Autodesk Inventor part; units mm, degrees
ref_plane "YZ Plane" through (0, 0, 0) normal (1, 0, 0) x (0, 1, 0)
ref_plane "XZ Plane" through (0, 0, 0) normal (0, 1, 0) x (-1, 0, 0)
ref_plane "XY Plane" through (0, 0, 0) normal (0, 0, 1) x (1, 0, 0)
sketch "Sketch1" plane through (0, 0, 0) normal (0, 1, 0) x (-1, 0, 0)
  line L0 (0, 0) -> (30, 0)
  line L1 (30, 0) -> (30, -150)
  line L2 (30, -150) -> (0, -150)
  line L3 (0, -150) -> (0, 0)
  dimension "d0" = 30
  dimension "d1" = 150
extrude "Extrusion1" add sketch "Sketch1" along normal blind 5
fillet "Fillet1" radius 15 4 edges at (0, 2.5, 0) (-30, 2.5, 0) (0, 2.5, -150) (-30, 2.5, -150)
sketch "Sketch2" plane through (0, 5, 0) normal (0, 1, 0) x (1, 0, 0)
  arc A0 (0, 135) -> (-30, 135) centre (-15, 135) ccw
  circle A1 centre (-15, 135) radius 5
  arc A2 (-30, 15) -> (0, 15) centre (-15, 15) ccw
  circle A3 centre (-15, 15) radius 5
  point P0 (0, 0)
  dimension "d5" = 10
  dimension "d6" = 10
extrude "Extrusion2" cut sketch "Sketch2" against normal blind 10
equation "\"d7\" = d6"
properties part number "Coupler Link"
Source: CAD feature listing. Evaluate the final solid. Frame: model axes, mm. Coordinates: 2 decimals unless noted, no trailing zeros. Loops run counter-clockwise (first coordinate to the right, second up) from the corner with the lowest first, then second, coordinate; pieces in that order, holes last. Notation, with made-up numbers: (57, 48) -> (75, 48) arc R10 ccw to (75, 57) -> close; hole circle Ø7 at (16.5, 79.5). An arc over 180 degrees is marked (long way). One line per item, written item: value. Start each with the question number.
Q1. Contact query for a flat-ended pin moving along its axis: P1, Ø2, axis at x = -11.5, y = 2, coming from the +Z side. Output: stop coordinate, or through.
Q2. Section query B-B, the plane x = -24.75. Return the cut outline in (y, z).
Q3. Line query: line 1 along X through (y, z) = (3.1, -135); line 2 along Z through (x, y) = (-16, 4.85); line 3 along Z through (x, y) = (-16.75, 3.95). Output: solid intervals per line, ascending.
Q4. Section query C-C, the plane x = -6. Return the cut outline in (y, z), and give its area (3 significant figures).
Q5. Section query A-A, the plane y = 2.1. Give the number of separate pieces and of enclosed holes in the cut face, and give its area (3 significant figures).
Q6. Mould query, pull axis X, two halves, no side actions, for faces 1 (the face through (-16.08, 2.54, -130.12)), 2 (the face through (-16.08, 2.54, -10.12)), 3 (the face through (-25.49, 2.54, -145.72)), 4 (the face through (-15, 0, -74)). Classes: pulls with the +X half, pulls with the -X half, needs draft (parallel to the pull), parting line crosses it, or undercut.
Results:
1. P1: z = -0.21
2. outline: (0, -146.4) -> (5, -146.4) -> (5, -3.6) -> (0, -3.6) -> close
3. line 1: -30 to -20, -10 to 0
3. line 2: -149.97 to -139.9, -130.1 to -19.9, -10.1 to -0.03
3. line 3: -149.9 to -139.68, -130.32 to -19.68, -10.32 to -0.1
4. outline: (0, -147) -> (5, -147) -> (5, -3) -> (0, -3) -> close
4. area: 720 mm^2
5. separate pieces: 1
5. enclosed holes: 2
5. area: 4,150 mm^2
6. face 1: undercut
6. face 2: undercut
6. face 3: pulls with the -X half
6. face 4: needs draft
